Check sheet for the modelled part. Datum: model origin and axes. Units: mm. Give positions to 0.01 mm unless a question says otherwise; leave off trailing zeros. Loops run counter-clockwise (first coordinate to the right, second up) from the corner with the lowest first, then second, coordinate; pieces in that order, holes last. Notation, with made-up numbers: M 45,36.25 L 76,36.25 A22 ccw 76,42.25 Z; hole C 47.25,88 d3. An arc over 180 degrees is marked long. Use one line per item in the form item = value.
from build123d import *

# Parameters (mm, degrees)
SKETCH_W        = 720
SKETCH_H        = 400
PAD_DEPTH       = 18
SKETCH001_W     = 9
SKETCH001_H     = 400
POCKET_DEPTH    = 9
SKETCH002_W     = 18
SKETCH002_H     = 400
POCKET001_DEPTH = 3.5


with BuildPart() as part:
    # Sketch → Pad (new body)
    with BuildSketch(Plane.XY):
        with Locations((-360, 200)):
            Rectangle(SKETCH_W, SKETCH_H)
    extrude(amount=PAD_DEPTH)

    # Sketch001 → Pocket (cut)
    with BuildSketch(Plane.XY):
        with Locations((-4.5, 200)):
            Rectangle(SKETCH001_W, SKETCH001_H)
        with Locations((-715.5, 200)):
            Rectangle(SKETCH001_W, SKETCH001_H)
    extrude(amount=POCKET_DEPTH, mode=Mode.SUBTRACT)

    # Sketch002 (on Face4 of Pocket) → Pocket001 (cut)
    with BuildSketch(Plane(origin=(0, 0, 0), x_dir=(1, 0, 0), z_dir=(0, 0, -1))):
        with Locations((-360, -200)):
            Rectangle(SKETCH002_W, SKETCH002_H)
    extrude(amount=-POCKET001_DEPTH, mode=Mode.SUBTRACT)


solid = part.part
1) Release check for a two-part mould opening along X. For faces 1 (the face through (-365, 203, 18)), 2 (the face through (-360, 197, 3.5)) record: pulls with the +X half, pulls with the -X half, needs draft (parallel to the pull), parting line crosses it, or undercut.
Evaluation:
face_1 = needs draft
face_2 = undercut
2) Scan lines: line 1 (X direction, y = 245.5, z = 2.5); line 2 (Z direction, x = -365.5, y = 172); line 3 (X direction, y = 101, z = 6). Record each from-to range of solid material in increasing order.
Evaluation:
line_1 = -711 to -369, -351 to -9
line_2 = 3.5 to 18
line_3 = -711 to -9
3) Depth check by flat-ended pin: pin 1 Ø1 at (y, z) = (273, 1) entering from -X; pin 2 Ø4.5 at (y, z) = (176.5, 4.5) entering from +X; pin 3 Ø4 at (y, z) = (120.5, 15.5) entering from +X; pin 4 Ø2.5 at (x, y) = (-716, 224.5) entering from -Z. Enter the tip coordinate at first touch or a pass-through.
Evaluation:
pin_1 = -711
pin_2 = -9
pin_3 = 0
pin_4 = 9
4) Section check A-A (y = 149). Record the cut outline in (x, z).
Evaluation:
outline = M -720,9 L -711,9 L -711,0 L -369,0 L -369,3.5 L -351,3.5 L -351,0 L -9,0 L -9,9 L 0,9 L 0,18 L -720,18 Z
